Here's how the part is built. I have some questions about the finished solid (model axes, mm). Coordinates: 2 decimals unless noted, no trailing zeros. Loops run counter-clockwise (first coordinate to the right, second up) from the corner with the lowest first, then second, coordinate; pieces in that order, holes last. Notation, with made-up numbers: (-39, -18.5) -> (15, -18.5) arc R10 ccw to (15, -0.5) -> close; hole circle Ø9 at (38, 78.25). An arc over 180 degrees is marked (long way). Answer as a JSON object with one key per item and string values. Group by question number.
Q1. I want a section at B-B on y = -621.5. Write out the boundary of the cut face in (x, z), then the cut area to 3 significant figures.
Q2. I want a section at C-C on x = 606. Write out the boundary of the cut face in (y, z).
Q3. I need wall thicknesses on line 1 (X direction, y = 22.5, z = 68.5); line 2 (X direction, y = -83, z = 21.5); line 3 (Y direction, x = 287.5, z = 35.5). Which ranges of each line are inside material? Lowest first, please.
Q4. I'm going to push a flat-ended pin straight in: pin 1 (24 mm diameter, centred on x = -44.39, z = 40, fed in from +Y). Where does the tip first touch, or does it pass through?
Q5. I want a section at A-A on z = 149. Write out the boundary of the cut face in (x, y).
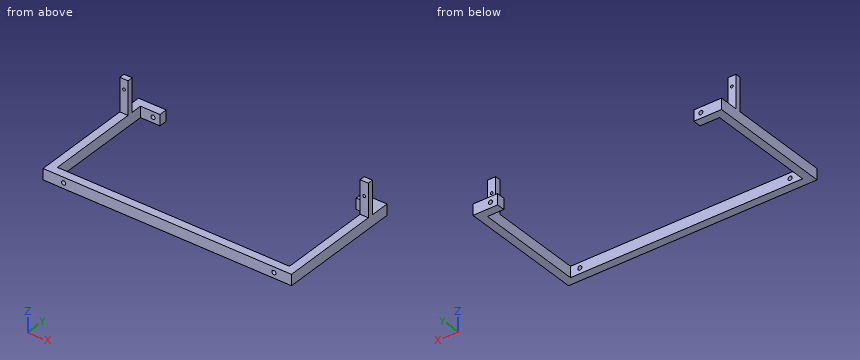
```python
from build123d import *

# Parameters (mm, degrees)
BOSS_EXTRU_1_DEPTH      = 80
ESQUISSE2_R             = 15
ENL_V_MAT_EXTRU_1_DEPTH = 1869.446312251
ESQUISSE3_W             = 60
ESQUISSE3_H             = 283.290811992
ESQUISSE3_R             = 10
BOSS_EXTRU_2_DEPTH      = 20


with BuildPart() as part:
    # Esquisse1 → Boss.-Extru.1 (new body)
    with BuildSketch(Plane.XY):
        Polygon((6.862464031, 0), (-135.71812121, 0), (-135.71812121, -800), (1564.28187879, -800), (1564.28187879, 0), (1444.276814416, 0), (1444.276814416, 60), (1624.28187879, 60), (1624.28187879, -860), (-195.71812121, -860), (-195.71812121, 60), (6.862464031, 60), align=None)
    extrude(amount=BOSS_EXTRU_1_DEPTH)

    # Esquisse2 → Enlèv. mat.-Extru.1 (cut, through all)
    with BuildSketch(Plane(origin=(0, 60, 0), x_dir=(1, 0, 0), z_dir=(0, 1, 0))):
        with Locations(Location((-44.394941641, -40, 0), (0, 0, 180))):
            Circle(ESQUISSE2_R)
        with Locations(Location((1495.605058359, -40, 0), (0, 0, 180))):
            Circle(ESQUISSE2_R)
    extrude(amount=-ENL_V_MAT_EXTRU_1_DEPTH, mode=Mode.SUBTRACT)

    # Esquisse3 → Boss.-Extru.2 (add, symmetric)
    # profile 1 of 2: a face of its own
    with BuildSketch(Plane(origin=(0, -100, 0), x_dir=(1, 0, 0), z_dir=(0, 1, 0))):
        with Locations((-165.71812121, -181.645405996)):
            Rectangle(ESQUISSE3_W, ESQUISSE3_H)
        with Locations(Location((-165.71812121, -250, 0), (0, 0, 270))):
            Circle(ESQUISSE3_R, mode=Mode.SUBTRACT)
    # profile 2 of 2: a face of its own
    with BuildSketch(Plane(origin=(0, -100, 0), x_dir=(1, 0, 0), z_dir=(0, 1, 0))):
        with Locations((1594.28187879, -181.645405996)):
            Rectangle(ESQUISSE3_W, ESQUISSE3_H)
        with Locations(Location((1594.28187879, -220, 0), (0, 0, 270))):
            Circle(ESQUISSE3_R, mode=Mode.SUBTRACT)
    extrude(amount=BOSS_EXTRU_2_DEPTH, both=True)


solid = part.part
```
Result set:
{
 "1": {"outline": "(-195.72, 0) -> (-135.72, 0) -> (-135.72, 80) -> (-195.72, 80) -> close; (1564.28, 0) -> (1624.28, 0) -> (1624.28, 80) -> (1564.28, 80) -> close", "area": "9,600 mm²"},
 "2": {"outline": "(-860, 0) -> (-800, 0) -> (-800, 80) -> (-860, 80) -> close"},
 "3": {"line 1": "x = -195.72 to 6.86, 1444.28 to 1624.28", "line 2": "x = -195.72 to -135.72, 1564.28 to 1624.28", "line 3": "y = -860 to -800"},
 "4": {"pin 1": "passes through"},
 "5": {"outline": "(-195.72, -120) -> (-135.72, -120) -> (-135.72, -80) -> (-195.72, -80) -> close; (1564.28, -120) -> (1624.28, -120) -> (1624.28, -80) -> (1564.28, -80) -> close"}
}
